from build123d import *

# Parameters (mm, degrees)
F0_W     = 18
F0_H     = 15.7
F1_DEPTH = 5.5
F2_R     = 0.5
F3_W     = 2
F3_H     = 2
F3_W_2   = 0.5
F4_DEPTH = 25
F3_W_3   = 13
F5_DEPTH = 2


with BuildPart() as f1:
    # F0 (on Top) → F1 (new body)
    with BuildSketch(Plane.XY):
        Rectangle(F0_W, F0_H)
    extrude(amount=-F1_DEPTH)

    # F2
    f2_edges = [f1.edges().sort_by_distance(p)[0] for p in [
        (9, 7.85, -2.75),
        (-9, 7.85, -2.75),
    ]]
    fillet(f2_edges, radius=F2_R)

    # F3 (on face) → F4 (cut)
    with BuildSketch(Plane(origin=(0, 7.85, 0), x_dir=(-1, 0, 0), z_dir=(0, 1, 0))):
        with Locations((-7.5, -2.9)):
            Rectangle(F3_W, F3_H)
        with Locations((-8.75, -2.9)):
            Rectangle(F3_W_2, F3_H)
        with Locations((7.5, -2.9)):
            Rectangle(F3_W, F3_H)
        with Locations((8.75, -2.9)):
            Rectangle(F3_W_2, F3_H)
    extrude(amount=-F4_DEPTH, mode=Mode.SUBTRACT)

    # F3 (on face) → F5 (cut)
    with BuildSketch(Plane(origin=(0, 7.85, 0), x_dir=(-1, 0, 0), z_dir=(0, 1, 0))):
        with Locations((0, -2.9)):
            Rectangle(F3_W_3, F3_H)
    extrude(amount=-F5_DEPTH, mode=Mode.SUBTRACT)


solid = f1.part
Verification items for the finished model (mm, model axes). A direction names the side the tool comes from. Give positions to 0.01 mm unless a question says otherwise; leave off trailing zeros. Loops run counter-clockwise (first coordinate to the right, second up) from the corner with the lowest first, then second, coordinate; pieces in that order, holes last.
1) Sectioned sample at A-A, the plane x = -7.5. Enter the section's corners in (y, z), then the cut area to 4 significant figures.
2) Thickness scan on line 1 along Z through (x, y) = (-7, 2.75); line 2 along X through (y, z) = (0, -3.05); line 3 along Y through (x, z) = (0.25, -2.65). Record the ranges inside material, lowest first.
3) Sectioned sample at D-D, the plane z = -2.3. Enter the section's corners in (x, y).
4) Depth check by flat-ended pin: pin 1 Ø1 at (y, z) = (-2.5, -3) entering from +X; pin 2 Ø1.6 at (y, z) = (-3, -3) entering from -X. Enter the tip coordinate at first touch or a pass-through.
5) Set-up check for faces 5 (the flat face through (9, 0, -5)), 6 (the flat face through (1, 6, -3.9)), 7 (the flat face through (-9, 0, -1)), 8 (the flat face through (6.5, -1, -3)), 9 (the flat face through (0, 5.85, -3)): record each of +Z, -Z, +X, -X, +Y, -Y from which the full face is reachable in a straight line by a thin tool's end or side.
6) Sectioned sample at B-B, the plane y = 4.75. Enter the section's corners in (x, z), then the cut area to 3 significant figures.
7) Sectioned sample at C-C, the plane x = -4. Enter the section's corners in (y, z), then the cut area to 4 significant figures.
8) Draft check along Z on faces 1 (the flat face through (-6.5, -1, -3)), 2 (the flat face through (0, 0, 0)), 3 (the flat face through (-1, 6, -1.9)), 4 (the flat face through (0, -7.85, -3)). Enter one of: pulls with the +Z half, pulls with the -Z half, needs draft (parallel to the pull), parting line crosses it, or undercut.
Answers:
1. outline: (-7.85, -5.5) - (7.85, -5.5) - (7.85, -3.9) - (-7.85, -3.9) - close; (-7.85, -1.9) - (7.85, -1.9) - (7.85, 0) - (-7.85, 0) - close
1. area: 54.95 mm2
2. line 1: z = -5.5 to -3.9, -1.9 to 0
2. line 2: x = -6.5 to 6.5
2. line 3: y = -7.85 to 5.85
3. outline: (-6.5, -7.85) - (6.5, -7.85) - (6.5, 5.85) - (-6.5, 5.85) - close
4. pin 1: stops at x = 6.5
4. pin 2: stops at x = -6.5
5. face 5: +Z, -Z, +X, +Y, -Y
5. face 6: +Y
5. face 7: +Z, -Z, -X, +Y, -Y
5. face 8: +X, +Y, -Y
5. face 9: +X, -X, +Y
6. outline: (-9, -5.5) - (9, -5.5) - (9, -3.9) - (6.5, -3.9) - (6.5, -1.9) - (9, -1.9) - (9, 0) - (-9, 0) - (-9, -1.9) - (-6.5, -1.9) - (-6.5, -3.9) - (-9, -3.9) - close
6. area: 89.0 mm2
7. outline: (-7.85, -5.5) - (7.85, -5.5) - (7.85, -3.9) - (5.85, -3.9) - (5.85, -1.9) - (7.85, -1.9) - (7.85, 0) - (-7.85, 0) - close
7. area: 82.35 mm2
8. face 1: undercut
8. face 2: pulls with the +Z half
8. face 3: undercut
8. face 4: needs draft
